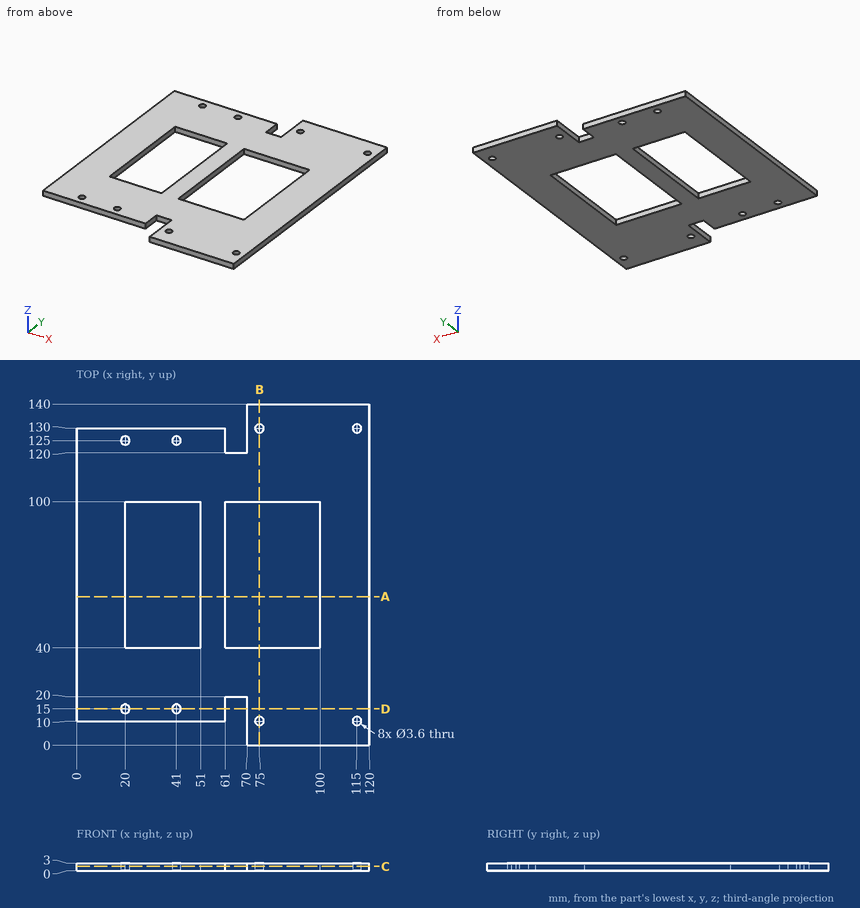
Geometry check sheet. Reference: drawing and pictorial views, mm from the part's lowest x, y, z. Give positions to 0.01 mm unless a question says otherwise; leave off trailing zeros. Order: outer loops, then holes, each group sorted by start corner. A loop starts at its lowest first (then second) coordinate and runs counter-clockwise, first axis right, second up. Notation, with made-up numbers: (16, 68.25) -> (54, 68.25) arc R23 cw to (54, 81.25) -> close; hole circle Ø7 at (-12, -8). An arc over 180 degrees is marked (long way). Use CSV: the item, a comma, the result in double quotes. Start each with the question number.
1) Sectioned sample at B-B, the plane x = 75. Record the boundary of the cut face in (y, z).
2) Go/stop test with flat-tipped pins: P1, Ø5, axis at x = 96.5, y = 44, coming from the +Z side; P2, Ø0.9, axis at x = 35, z = 1.5, coming from the +Y side; P3, Ø1.5, axis at x = 63.5, z = 1, coming from the -Y side; P4, Ø0.9, axis at x = 22, z = 1, coming from the -Y side. Record where each tip stops, or that it passes through.
3) Sectioned sample at C-C, the plane z = 1.8. Give the number of separate pieces and of enclosed holes in the cut face, plus the area to 3 significant figures.
4) Sectioned sample at D-D, the plane y = 15. Record the boundary of the cut face in (x, z).
5) Material ranges on line 1 (Y direction, x = 115, z = 0.6); line 2 (X direction, y = 95.5, z = 2.5); line 3 (Y direction, x = 75, z = 1.7), recorded low to high. Write a range as from..to.
6) Sectioned sample at A-A, the plane y = 61. Record the boundary of the cut face in (x, z).
Recorded:
1,outline,"(0, 0) -> (8.2, 0) -> (8.2, 3) -> (0, 3) -> close; (11.8, 0) -> (40, 0) -> (40, 3) -> (11.8, 3) -> close; (100, 0) -> (128.2, 0) -> (128.2, 3) -> (100, 3) -> close; (131.8, 0) -> (140, 0) -> (140, 3) -> (131.8, 3) -> close"
2,P1,"through"
2,P2,"y = 130"
2,P3,"y = 20"
2,P4,"y = 10"
3,separate pieces,"1"
3,enclosed holes,"10"
3,area,"10,900 mm2"
4,outline,"(0, 0) -> (18.2, 0) -> (18.2, 3) -> (0, 3) -> close; (21.8, 0) -> (39.2, 0) -> (39.2, 3) -> (21.8, 3) -> close; (42.8, 0) -> (61, 0) -> (61, 3) -> (42.8, 3) -> close; (70, 0) -> (120, 0) -> (120, 3) -> (70, 3) -> close"
5,line 1,"0..8.2, 11.8..128.2, 131.8..140"
5,line 2,"0..20, 51..61, 100..120"
5,line 3,"0..8.2, 11.8..40, 100..128.2, 131.8..140"
6,outline,"(0, 0) -> (20, 0) -> (20, 3) -> (0, 3) -> close; (51, 0) -> (61, 0) -> (61, 3) -> (51, 3) -> close; (100, 0) -> (120, 0) -> (120, 3) -> (100, 3) -> close"
